```python
from build123d import *

# Parameters (mm, degrees)
F0_R     = 4.6
F0_R_2   = 1.5
F1_DEPTH = 3


with BuildPart() as f1:
    # F0 (on Front) → F1 (new body)
    with BuildSketch(Plane.XZ):
        with BuildLine():
            ThreePointArc((24.286818, 36.347792), (18.751488, 45.270097), (8.528396, 42.875144))
            ThreePointArc((8.528396, 42.875144), (0, 49), (-8.528396, 42.875144))
            ThreePointArc((-8.528396, 42.875144), (-18.751488, 45.270097), (-24.286818, 36.347792))
            ThreePointArc((-24.286818, 36.347792), (-34.648232, 34.648232), (-36.347792, 24.286818))
            ThreePointArc((-36.347792, 24.286818), (-45.270097, 18.751488), (-42.875144, 8.528396))
            ThreePointArc((-42.875144, 8.528396), (-49, 0), (-42.875144, -8.528396))
            ThreePointArc((-42.875144, -8.528396), (-45.270097, -18.751488), (-36.347792, -24.286818))
            ThreePointArc((-36.347792, -24.286818), (-34.648232, -34.648232), (-24.286818, -36.347792))
            ThreePointArc((-24.286818, -36.347792), (-18.751488, -45.270097), (-8.528396, -42.875144))
            ThreePointArc((-8.528396, -42.875144), (0, -49), (8.528396, -42.875144))
            ThreePointArc((8.528396, -42.875144), (18.751488, -45.270097), (24.286818, -36.347792))
            ThreePointArc((24.286818, -36.347792), (34.648232, -34.648232), (36.347792, -24.286818))
            ThreePointArc((36.347792, -24.286818), (45.270097, -18.751488), (42.875144, -8.528396))
            ThreePointArc((42.875144, -8.528396), (49, 0), (42.875144, 8.528396))
            ThreePointArc((42.875144, 8.528396), (45.270097, 18.751488), (36.347792, 24.286818))
            ThreePointArc((36.347792, 24.286818), (34.648232, 34.648232), (24.286818, 36.347792))
        make_face()
        with Locations((-28.284271, -28.284271)):
            Circle(F0_R, mode=Mode.SUBTRACT)
        with Locations((-15.307337, -36.955181)):
            Circle(F0_R, mode=Mode.SUBTRACT)
        with Locations((0, -40)):
            Circle(F0_R, mode=Mode.SUBTRACT)
        with Locations((0, -27)):
            Circle(F0_R_2, mode=Mode.SUBTRACT)
        with Locations((-36.955181, -15.307337)):
            Circle(F0_R, mode=Mode.SUBTRACT)
        with Locations((-40, 0)):
            Circle(F0_R, mode=Mode.SUBTRACT)
        with Locations((-27, 0)):
            Circle(F0_R_2, mode=Mode.SUBTRACT)
        with BuildLine():
            ThreePointArc((-2.145994, 10.788638), (0, 11), (2.145994, 10.788638))
            ThreePointArc((2.145994, 10.788638), (4.209518, 10.162675), (6.111273, 9.146166))
            ThreePointArc((6.111273, 9.146166), (7.778175, 7.778175), (9.146166, 6.111273))
            ThreePointArc((9.146166, 6.111273), (10.162675, 4.209518), (10.788638, 2.145994))
            ThreePointArc((10.788638, 2.145994), (11, 0), (10.788638, -2.145994))
            ThreePointArc((10.788638, -2.145994), (10.162675, -4.209518), (9.146166, -6.111273))
            ThreePointArc((9.146166, -6.111273), (7.778175, -7.778175), (6.111273, -9.146166))
            ThreePointArc((6.111273, -9.146166), (4.209518, -10.162675), (2.145994, -10.788638))
            ThreePointArc((2.145994, -10.788638), (0, -11), (-2.145994, -10.788638))
            ThreePointArc((-2.145994, -10.788638), (-4.209518, -10.162675), (-6.111273, -9.146166))
            ThreePointArc((-6.111273, -9.146166), (-7.778175, -7.778175), (-9.146166, -6.111273))
            ThreePointArc((-9.146166, -6.111273), (-10.162675, -4.209518), (-10.788638, -2.145994))
            ThreePointArc((-10.788638, -2.145994), (-11, 0), (-10.788638, 2.145994))
            ThreePointArc((-10.788638, 2.145994), (-10.162675, 4.209518), (-9.146166, 6.111273))
            ThreePointArc((-9.146166, 6.111273), (-7.778175, 7.778175), (-6.111273, 9.146166))
            ThreePointArc((-6.111273, 9.146166), (-4.209518, 10.162675), (-2.145994, 10.788638))
        make_face(mode=Mode.SUBTRACT)
        with Locations((15.307337, -36.955181)):
            Circle(F0_R, mode=Mode.SUBTRACT)
        with Locations((28.284271, -28.284271)):
            Circle(F0_R, mode=Mode.SUBTRACT)
        with Locations((36.955181, -15.307337)):
            Circle(F0_R, mode=Mode.SUBTRACT)
        with Locations((27, 0)):
            Circle(F0_R_2, mode=Mode.SUBTRACT)
        with Locations((40, 0)):
            Circle(F0_R, mode=Mode.SUBTRACT)
        with Locations((-36.955181, 15.307337)):
            Circle(F0_R, mode=Mode.SUBTRACT)
        with Locations((-28.284271, 28.284271)):
            Circle(F0_R, mode=Mode.SUBTRACT)
        with Locations((0, 27)):
            Circle(F0_R_2, mode=Mode.SUBTRACT)
        with Locations((-15.307337, 36.955181)):
            Circle(F0_R, mode=Mode.SUBTRACT)
        with Locations((0, 40)):
            Circle(F0_R, mode=Mode.SUBTRACT)
        with Locations((36.955181, 15.307337)):
            Circle(F0_R, mode=Mode.SUBTRACT)
        with Locations((15.307337, 36.955181)):
            Circle(F0_R, mode=Mode.SUBTRACT)
        with Locations((28.284271, 28.284271)):
            Circle(F0_R, mode=Mode.SUBTRACT)
    extrude(amount=F1_DEPTH)


solid = f1.part
```
The listing builds one solid part. Answer for the finished solid, in the listing's coordinates (mm). Give positions to 0.01 mm unless a question says otherwise; leave off trailing zeros. Order: outer loops, then holes, each group sorted by start corner. A loop starts at its lowest first (then second) coordinate and runs counter-clockwise, first axis right, second up. Notation, with made-up numbers: (89.25, 78) -> (105.25, 78) arc R20 ccw to (105.25, 99) -> close; hole circle Ø9 at (63.5, -39). An arc over 180 degrees is marked (long way). Answer as CSV lines item,"result". Start each with the question number.
Q1. Find the intervals of material crossed by L1, parallel to Z at x = 34, y = -1; L2, parallel to X at y = -1.7, z = -2, in increasing order.
Q2. A cutting plane is placed at A-A (z = 0). Determine the outline of the cut face in (x, y).
Q3. A cutting plane is placed at C-C (x = 40). Determine the outline of the cut face in (y, z).
Q4. Given pin 1 (1 mm diameter, centred on x = -12, y = -1.5, fed in from +Z), flat-ended and moving along its own axis, determine where the tip first touches the part or whether it passes through.
Q5. Determine the mould class of faces 1 (the cylindrical face through (-28.5, -1.48, 0.07)), 2 (the flat face through (-1, 0, 12)) for opening direction X: pulls with the +X half, pulls with the -X half, needs draft (parallel to the pull), parting line crosses it, or undercut.
Q6. A cutting plane is placed at D-D (z = 13.5). Determine the outline of the cut face in (x, y).
Q7. A cutting plane is placed at B-B (x = 18.5). Determine the outline of the cut face in (y, z).
Results found:
1,L1,"-35.24 to -18.83, -11.78 to 11.78, 18.83 to 35.24"
1,L2,"-48.77 to -44.14, -35.86 to -10.82, 10.82 to 35.86, 44.14 to 48.77"
2,outline,"(-49, -3) -> (-44.6, -3) -> (-44.6, 0) -> (-49, 0) -> close; (-35.4, -3) -> (-28.5, -3) -> (-28.5, 0) -> (-35.4, 0) -> close; (-25.5, -3) -> (-11, -3) -> (-11, 0) -> (-25.5, 0) -> close; (11, -3) -> (25.5, -3) -> (25.5, 0) -> (11, 0) -> close; (28.5, -3) -> (35.4, -3) -> (35.4, 0) -> (28.5, 0) -> close; (44.6, -3) -> (49, -3) -> (49, 0) -> (44.6, 0) -> close"
3,outline,"(-3, -23.78) -> (0, -23.78) -> (0, -18.76) -> (-3, -18.76) -> close; (-3, -11.86) -> (0, -11.86) -> (0, -4.6) -> (-3, -4.6) -> close; (-3, 4.6) -> (0, 4.6) -> (0, 11.86) -> (-3, 11.86) -> close; (-3, 18.76) -> (0, 18.76) -> (0, 23.78) -> (-3, 23.78) -> close"
4,pin 1,"z = 45.51"
5,face 1,"undercut"
5,face 2,"needs draft"
6,outline,"(-45.77, -3) -> (-41.19, -3) -> (-41.19, 0) -> (-45.77, 0) -> close; (-32.73, -3) -> (32.73, -3) -> (32.73, 0) -> (-32.73, 0) -> close; (41.19, -3) -> (45.77, -3) -> (45.77, 0) -> (41.19, 0) -> close"
7,outline,"(-3, -45.37) -> (0, -45.37) -> (0, -40.27) -> (-3, -40.27) -> close; (-3, -33.64) -> (0, -33.64) -> (0, 33.64) -> (-3, 33.64) -> close; (-3, 40.27) -> (0, 40.27) -> (0, 45.37) -> (-3, 45.37) -> close"
